The figure shows three views and two pictorial views of one solid part (mm, origin at its lowest corner). Answer the questions. A direction names the side the tool comes from. Round coordinates to 2 decimals unless told otherwise and drop trailing zeros. Order: outer loops, then holes, each group sorted by start corner. A loop starts at its lowest first (then second) coordinate and runs counter-clockwise, first axis right, second up. Notation, with made-up numbers: (-21.75, -12) - (11.25, -12) arc R17 ccw to (11.25, -3) - close; hole circle Ø7 at (70.25, 26). An arc over 180 degrees is marked (long way). Use CSV: the item, a comma, the result in double quotes. Start each with the question number.
Item 1: Straight lines are drawn through the part: line 1 along Y through (x, z) = (6.1, 13.15); line 2 along Z through (x, y) = (5, 14); line 3 along Z through (x, y) = (4.25, 19). For each, find the intervals that lie inside material, in ascending order. Write a range as [from, to].
Item 2: Find section D-D, the plane y = 10.6. Give the vertices of the cut face in (x, z).
Item 3: Flat-ended cylindrical pins translate along their axes: P1, Ø1.6, axis at x = 6.1, y = 2.3, coming from the +Z side; P2, Ø2, axis at x = 7.5, z = 18, coming from the +Y side; P3, Ø4, axis at x = 4, y = 2.5, coming from the -Z side; P4, Ø4, axis at x = 6.5, y = 31, coming from the +Z side. Find the tip coordinate at first contact, or state that the pin passes through.
Item 4: Find section C-C, the plane x = 1.5. Give the vertices of the cut face in (y, z).
Item 5: Find section A-A, the plane y = 2.3. Give the vertices of the cut face in (x, z).
Item 6: For the marked faces 1, 2 and 3, determine the directions among +Z, -Z, +X, -X, +Y, -Y from which every point of the face is accessible in a straight line to the end or side of a thin tool.
Item 7: Determine the mould class of the marked faces 4, 5 and 6 for opening direction Z: +Z half, -Z half, draft (parallel to the pull), parting line (faces both ways), or undercut.
Item 8: Find section B-B, the plane z = 14.5. Give the vertices of the cut face in (x, y), plus the area to 3 significant figures.
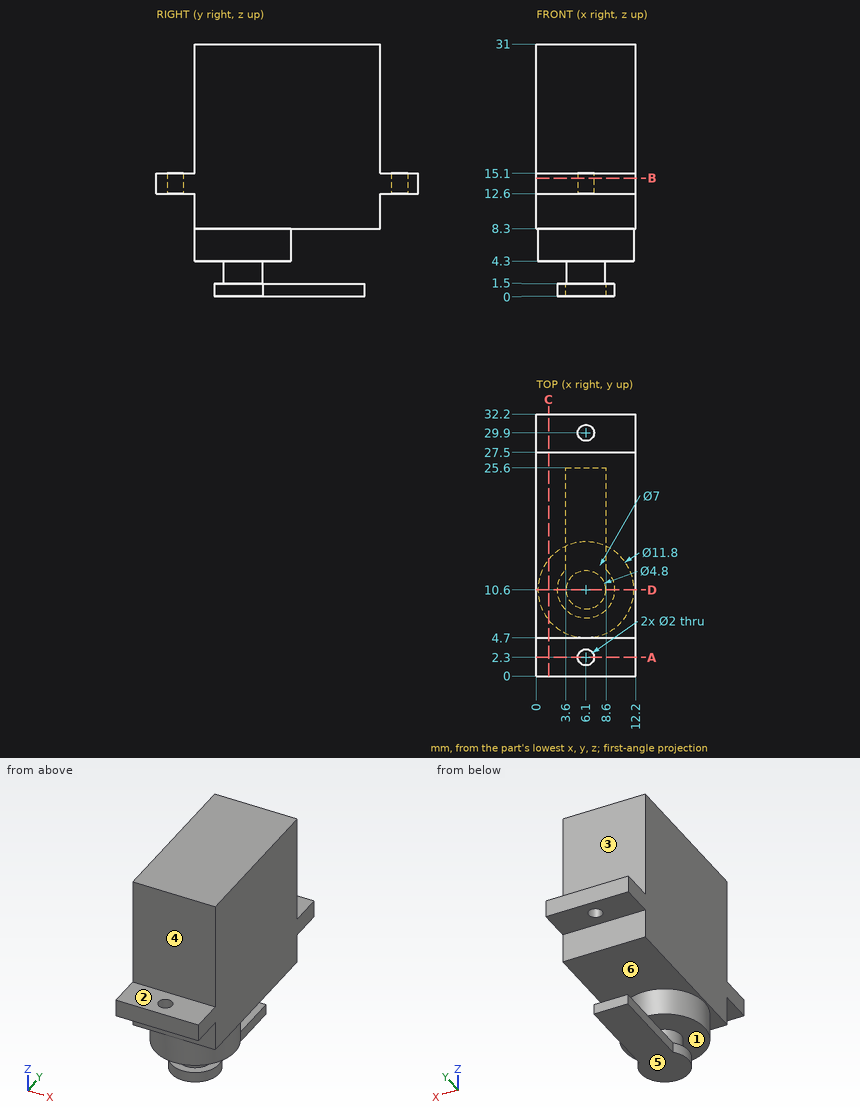
Worked out:
1,line 1,"y = [0, 1.3], [3.3, 28.9], [30.9, 32.2]"
1,line 2,"z = [0, 1.5], [4.3, 31]"
1,line 3,"z = [0, 1.5], [8.3, 31]"
2,outline,"(0, 8.3) - (0.2, 8.3) - (0.2, 4.3) - (3.7, 4.3) - (3.7, 1.5) - (2.6, 1.5) - (2.6, 0) - (9.6, 0) - (9.6, 1.5) - (8.5, 1.5) - (8.5, 4.3) - (12, 4.3) - (12, 8.3) - (12.2, 8.3) - (12.2, 31) - (0, 31) - close"
3,P1,"passes through"
3,P2,"stops at y = 27.5"
3,P3,"stops at z = 12.6"
3,P4,"stops at z = 15.1"
4,outline,"(0, 12.6) - (4.7, 12.6) - (4.7, 8.3) - (6.91, 8.3) - (6.91, 4.3) - (14.29, 4.3) - (14.29, 8.3) - (27.5, 8.3) - (27.5, 12.6) - (32.2, 12.6) - (32.2, 15.1) - (27.5, 15.1) - (27.5, 31) - (4.7, 31) - (4.7, 15.1) - (0, 15.1) - close"
5,outline,"(0, 12.6) - (5.1, 12.6) - (5.1, 15.1) - (0, 15.1) - close; (7.1, 12.6) - (12.2, 12.6) - (12.2, 15.1) - (7.1, 15.1) - close"
6,face 1,"none"
6,face 2,"+Z, +X, -X, -Y"
6,face 3,"+Z, +X, -X, +Y"
7,face 4,"draft"
7,face 5,"-Z half"
7,face 6,"undercut"
8,outline,"(0, 0) - (12.2, 0) - (12.2, 32.2) - (0, 32.2) - close; hole circle Ø2 at (6.1, 2.3); hole circle Ø2 at (6.1, 29.9)"
8,area,"387 mm²"
